```python
from build123d import *

# Parameters (mm, degrees)
SKETCH_1_R          = 45
EXTRUDE_1_DEPTH     = 25
SKETCH_2_R          = 12.5
CUT_EXTRUDE_2_DEPTH = 69.373971656
SKETCH_3_R          = 30
CUT_EXTRUDE_3_DEPTH = 20
SKETCH_4_R          = 2.5
CUT_EXTRUDE_4_DEPTH = 69.373971656
SKETCH_6_R          = 6
CUT_EXTRUDE_5_DEPTH = 5.5


with BuildPart() as part:
    # Эскиз1 → Вытянуть1 (new body)
    with BuildSketch(Plane.XY):
        Circle(SKETCH_1_R)
    extrude(amount=EXTRUDE_1_DEPTH)

    # Эскиз2 → Вытянуть2 (cut, through all)
    with BuildSketch(Plane.XY.offset(25)):
        Circle(SKETCH_2_R)
    extrude(amount=-CUT_EXTRUDE_2_DEPTH, mode=Mode.SUBTRACT)

    # Эскиз3 → Вытянуть3 (cut)
    with BuildSketch(Plane(origin=(0, 0, 0), x_dir=(-1, 0, 0), z_dir=(0, 0, -1))):
        Circle(SKETCH_3_R)
    extrude(amount=-CUT_EXTRUDE_3_DEPTH, mode=Mode.SUBTRACT)

    # Эскиз4 → Вытянуть4 (cut, through all)
    with BuildSketch(Plane.XY.offset(25)):
        with Locations((0, 37.683516186)):
            Circle(SKETCH_4_R)
        with Locations((26.646269834, 26.646269834)):
            Circle(SKETCH_4_R)
        with Locations((37.683516186, 0)):
            Circle(SKETCH_4_R)
        with Locations((26.646269834, -26.646269834)):
            Circle(SKETCH_4_R)
        with Locations((0, -37.683516186)):
            Circle(SKETCH_4_R)
        with Locations((-26.646269834, -26.646269834)):
            Circle(SKETCH_4_R)
        with Locations((-37.683516186, 0)):
            Circle(SKETCH_4_R)
        with Locations((-26.646269834, 26.646269834)):
            Circle(SKETCH_4_R)
    extrude(amount=-CUT_EXTRUDE_4_DEPTH, mode=Mode.SUBTRACT)

    # Эскиз6 → Вытянуть5 (cut)
    with BuildSketch(Plane.XY.offset(25)):
        with Locations((0, 37.683516186)):
            Circle(SKETCH_6_R)
        with Locations((26.646269834, 26.646269834)):
            Circle(SKETCH_6_R)
        with Locations((37.683516186, 0)):
            Circle(SKETCH_6_R)
        with Locations((26.646269834, -26.646269834)):
            Circle(SKETCH_6_R)
        with Locations((0, -37.683516186)):
            Circle(SKETCH_6_R)
        with Locations((-26.646269834, -26.646269834)):
            Circle(SKETCH_6_R)
        with Locations((-37.683516186, 0)):
            Circle(SKETCH_6_R)
        with Locations((-26.646269834, 26.646269834)):
            Circle(SKETCH_6_R)
    extrude(amount=-CUT_EXTRUDE_5_DEPTH, mode=Mode.SUBTRACT)


solid = part.part
```
Check sheet for the modelled part. Datum: model origin and axes. Units: mm. A direction names the side the tool comes from. Coordinates: 2 decimals unless noted, no trailing zeros. Order: outer loops, then holes, each group sorted by start corner. A loop starts at its lowest first (then second) coordinate and runs counter-clockwise, first axis right, second up. Notation, with made-up numbers: (49.5, -35.5) -> (81.5, -35.5) arc R16 ccw to (81.5, -25.5) -> close; hole circle Ø9 at (6.5, -24.75). An arc over 180 degrees is marked (long way). Write item = value, one per line. Start each with the question number.
1) Mould release check, pull along Y, two halves, no side actions. Record for faces 1 (the flat face through (9, -9, 25)), 2 (the cylindrical face through (20.765, -39.923, 12.325)), 3 (the cylindrical face through (1.344, -35.576, 9.886)), 4 (the flat face through (-13, 0, 20)): +Y half, -Y half, draft (parallel to the pull), parting line (faces both ways), or undercut.
2) Material ranges on L1, parallel to Y at x = 0, z = 21.4; L2, parallel to X at y = 24.5, z = 5.5; L3, parallel to X at y = -28.5, z = 23.75, recorded low to high.
3) Cross-section at C-C (z = 22.5). State how many separate pieces and enclosed holes the cut face has, then the cut area to 3 significant figures.
4) Cross-section at D-D (x = -9). Enter the section's corners in (y, z), then the cut area to 3 significant figures.
5) Cross-section at A-A (x = 0). Enter the section's corners in (y, z), then the cut area to 3 significant figures.
6) Access from +Z, -Z, +X, -X, +Y, -Y to the whole of each face (thin tool, end or side, straight path). Record for faces 5 (the cylindrical face through (-25.302, 28.754, 9.886)), 6 (the cylindrical face through (31.69, 0.26, 22.29)), 7 (the cylindrical face through (29.97, 1.32, 9.86)).
7) Go/stop test with flat-tipped pins: P1, Ø9.5, axis at x = -37.68, y = 0, coming from the -Z side; P2, Ø3, axis at x = 12, z = 3, coming from the +Y side; P3, Ø4, axis at x = 26.65, y = -26.65, coming from the +Z side; P4, Ø2, axis at y = 7.5, z = 21, coming from the +X side. Record where each tip stops, or that it passes through.
Ans:
q1.face_1 = draft
q1.face_2 = parting line
q1.face_3 = undercut
q1.face_4 = undercut
q2.L1 = -45 to -43.68, -31.68 to -12.5, 12.5 to 31.68, 43.68 to 45
q2.L2 = -37.75 to -27.93, -25.36 to -17.31, 17.31 to 25.36, 27.93 to 37.75
q2.L3 = -34.82 to -32.35, -20.94 to 20.94, 32.35 to 34.82
q3.separate_pieces = 1
q3.enclosed_holes = 9
q3.area = 4,970 mm²
q4.outline = (-44.09, 0) -> (-28.62, 0) -> (-28.62, 20) -> (-8.67, 20) -> (-8.67, 25) -> (-44.09, 25) -> close; (8.67, 20) -> (28.62, 20) -> (28.62, 0) -> (44.09, 0) -> (44.09, 25) -> (8.67, 25) -> close
q4.area = 973 mm²
q5.outline = (-45, 0) -> (-40.18, 0) -> (-40.18, 19.5) -> (-43.68, 19.5) -> (-43.68, 25) -> (-45, 25) -> close; (-35.18, 0) -> (-30, 0) -> (-30, 20) -> (-12.5, 20) -> (-12.5, 25) -> (-31.68, 25) -> (-31.68, 19.5) -> (-35.18, 19.5) -> close; (12.5, 20) -> (30, 20) -> (30, 0) -> (35.18, 0) -> (35.18, 19.5) -> (31.68, 19.5) -> (31.68, 25) -> (12.5, 25) -> close; (40.18, 0) -> (45, 0) -> (45, 25) -> (43.68, 25) -> (43.68, 19.5) -> (40.18, 19.5) -> close
q5.area = 598 mm²
q6.face_5 = +Z, -Z
q6.face_6 = +Z
q6.face_7 = -Z
q7.P1 = 0
q7.P2 = 43.76
q7.P3 = through
q7.P4 = 44.53
